Read the model definition and answer for the solid it produces. Units are mm, in the model's axes. A direction names the side the tool comes from. Coordinates: 2 decimals unless noted, no trailing zeros. Loops run counter-clockwise (first coordinate to the right, second up) from the corner with the lowest first, then second, coordinate; pieces in that order, holes last. Notation, with made-up numbers: (-23, 10) -> (20, 10) arc R16 ccw to (20, 34) -> close; hole circle Ø1 at (62, 82.25). An arc over 180 degrees is marked (long way). Answer as a JSON object with one key per item and string values. Group by question number.
Q1. The part is cut by section D-D on x = 27. Write down the section's boundary in (y, z).
Q2. For faces 1 (the cylindrical face through (12.65, 3.84, 2)), 2 (the cylindrical face through (2.024, 3.609, -4.707)), determine the directions among +Z, -Z, +X, -X, +Y, -Y from which every point of the face is accessible in a straight line to the end or side of a thin tool.
Q3. The part is cut by section C-C on x = 8. Write down the section's boundary in (y, z).
Q4. Straight lines are drawn through the part: line 1 along Z through (x, y) = (11, -0.25); line 2 along Y through (x, z) = (16.5, 3); line 3 along Z through (x, y) = (10, -3.25). For each, find the intervals that lie inside material, in ascending order. Write a range as [from, to].
Q5. Each of these flat-tipped pins is pushed along its axis until it touches: P1, Ø4, axis at x = 30, z = 4, coming from the +Y side; P2, Ø1, axis at x = 21.5, y = 0.5, coming from the +Z side; P3, Ø6, axis at y = -3, z = 1.5, coming from the +X side; P4, Ø5, axis at x = 13.5, z = 2, coming from the -Y side. Where does it stop, or does it pass through?
from build123d import *


with BuildPart() as part:
    # Sketch1 → Revolve2 (revolve)
    with BuildSketch(Plane.XY, mode=Mode.PRIVATE) as revolve2_sk:
        with BuildLine():
            Line((1.496304491, 5.9309), (1.496304491, 0))
            Line((1.496304491, 0), (31.087304489, 0))
            Line((31.087304489, 0), (31.658804491, 0))
            Line((31.658804491, 0), (32.230304494, 0))
            Line((32.230304494, 0), (33.246304491, 0))
            ThreePointArc((33.246304491, 0), (32.781336507, 1.122532015), (31.658804491, 1.5875))
            Line((31.658804491, 1.5875), (31.021091308, 1.5875))
            ThreePointArc((31.021091308, 1.5875), (25.663749675, 2.239020867), (20.618721916, 4.155602128))
            ThreePointArc((20.618721916, 4.155602128), (20.27474275, 4.286278123), (19.909469457, 4.3307))
            Line((19.909469457, 4.3307), (5.594648416, 4.3307))
            Line((5.594648416, 4.3307), (2.940913387, 5.83211104))
            ThreePointArc((2.940913387, 5.83211104), (2.759693318, 5.905789005), (2.565686634, 5.9309))
            Line((2.565686634, 5.9309), (1.496304491, 5.9309))
        make_face()
    revolve(revolve2_sk.sketch.rotate(Axis((0, 0, 0), (1, 0, 0)), 90), axis=Axis((0, 0, 0), (1, 0, 0)))  # turned: the seam where the file's is


solid = part.part
Final values:
{
 "1": {"outline": "circle Ø3.9 at (0, 0)"},
 "2": {"face 1": "+X", "face 2": "+X, -X"},
 "3": {"outline": "circle Ø8.66 at (0, 0)"},
 "4": {"line 1": "z = [-4.32, 4.32]", "line 2": "y = [-3.12, 3.12]", "line 3": "z = [-2.86, 2.86]"},
 "5": {"P1": "passes through", "P2": "stops at z = 3.93", "P3": "stops at x = 33.21", "P4": "stops at y = -4.33"}
}
